The listing builds one solid part. Answer for the finished solid, in the listing's coordinates (mm). Face numbers are marked on the shaded views. Coordinates: 2 decimals unless noted, no trailing zeros. Order: outer loops, then holes, each group sorted by start corner. A loop starts at its lowest first (then second) coordinate and runs counter-clockwise, first axis right, second up. Notation, with made-up numbers: (-13, 78.5) - (42, 78.5) arc R17 cw to (42, 95.5) - close; hole circle Ø9 at (47, 11). An arc over 180 degrees is marked (long way). Use a Markdown table: item, result. Add a question column.
Item 1: The part is cut by section C-C, the plane y = 3.9. Give the vertices of the cut face in (x, z).
Item 2: The part is cut by section D-D, the plane x = -13.5. Give the vertices of the cut face in (y, z).
Item 3: Find the intervals of material crossed by line 1 along Y through (x, z) = (13, -1.75); line 2 along X through (y, z) = (4.85, 1); line 3 along Z through (x, y) = (1.5, 2.15), in increasing order.
Item 4: The mould has two halves that part along Z. Classify the marked faces 1, 2 and 3: released by +Z, released by -Z, zero draft, split by the parting line, or undercut.
Item 5: The part is cut by section A-A, the plane y = 1.5. State how many separate pieces and enclosed holes the cut face has, then the cut area to 3 significant figures.
Item 6: Flat-ended cylindrical pins translate along their axes: P1, Ø3, axis at x = -7.5, z = 0, coming from the -Y side; P2, Ø2.5, axis at x = 7.5, z = 0, coming from the +Y side; P3, Ø3, axis at y = 1.5, z = 2, coming from the +X side. Find the tip coordinate at first contact, or state that the pin passes through.
Item 7: The part is cut by section B-B, the plane x = 0. Give the vertices of the cut face in (y, z), then the cut area to 3 significant figures.
from build123d import *

# Parameters (mm, degrees)
BOSS_EXTRUDE1_DEPTH = 2
SKETCH2_R           = 4
SKETCH2_R_2         = 2.5
BOSS_EXTRUDE2_DEPTH = 3.5
SKETCH3_R           = 1.5
CUT_EXTRUDE1_DEPTH  = 5
SKETCH4_R           = 3
CUT_EXTRUDE2_DEPTH  = 1
SKETCH5_R           = 1
CUT_EXTRUDE3_DEPTH  = 5


with BuildPart() as part:
    # Sketch1 → Boss-Extrude1 (new body)
    with BuildSketch(Plane(origin=(0, 0, 0), x_dir=(1, 0, 0), z_dir=(0, 1, 0))):
        with BuildLine():
            Line((-16.5, 2.5), (-4.472135955, 4))
            ThreePointArc((-4.472135955, 4), (0, 6), (4.472135955, 4))
            Line((4.472135955, 4), (16.5, 2.5))
            ThreePointArc((16.5, 2.5), (19, 0), (16.5, -2.5))
            Line((16.5, -2.5), (4.472135955, -4))
            ThreePointArc((4.472135955, -4), (0, -6), (-4.472135955, -4))
            Line((-4.472135955, -4), (-16.5, -2.5))
            ThreePointArc((-16.5, -2.5), (-19, 0), (-16.5, 2.5))
        make_face()
    extrude(amount=BOSS_EXTRUDE1_DEPTH)

    # Sketch2 → Boss-Extrude2 (add)
    with BuildSketch(Plane(origin=(0, 2, 0), x_dir=(1, 0, 0), z_dir=(0, 1, 0))):
        with Locations(Location((0, 0, 0), (0, 0, 270))):
            Circle(SKETCH2_R)
        with Locations(Location((0, 0, 0), (0, 0, 270))):
            Circle(SKETCH2_R_2, mode=Mode.SUBTRACT)
    extrude(amount=BOSS_EXTRUDE2_DEPTH)

    # Sketch3 → Cut-Extrude1 (cut)
    with BuildSketch(Plane(origin=(0, 2, 0), x_dir=(1, 0, 0), z_dir=(0, 1, 0))):
        with Locations(Location((0, 0, 0), (0, 0, 270))):
            Circle(SKETCH3_R)
    extrude(amount=-CUT_EXTRUDE1_DEPTH, mode=Mode.SUBTRACT)

    # Sketch4 → Cut-Extrude2 (cut)
    with BuildSketch(Plane.XZ):
        with Locations(Location((0, 0, 0), (0, 0, 270))):
            Circle(SKETCH4_R)
    extrude(amount=-CUT_EXTRUDE2_DEPTH, mode=Mode.SUBTRACT)

    # Sketch5 → Cut-Extrude3 (cut)
    with BuildSketch(Plane.XZ):
        with Locations(Location((-16.5, 0, 0), (0, 0, 270))):
            Circle(SKETCH5_R)
        with Locations(Location((-10.5, 0, 0), (0, 0, 270))):
            Circle(SKETCH5_R)
        with Locations(Location((-7.5, 0, 0), (0, 0, 270))):
            Circle(SKETCH5_R)
        with Locations(Location((7.5, 0, 0), (0, 0, 270))):
            Circle(SKETCH5_R)
        with Locations(Location((10.5, 0, 0), (0, 0, 270))):
            Circle(SKETCH5_R)
        with Locations(Location((13.5, 0, 0), (0, 0, 270))):
            Circle(SKETCH5_R)
        with Locations(Location((16.5, 0, 0), (0, 0, 270))):
            Circle(SKETCH5_R)
        with Locations(Location((-13.5, 0, 0), (0, 0, 90))):
            Circle(SKETCH5_R)
    extrude(amount=-CUT_EXTRUDE3_DEPTH, mode=Mode.SUBTRACT)


solid = part.part
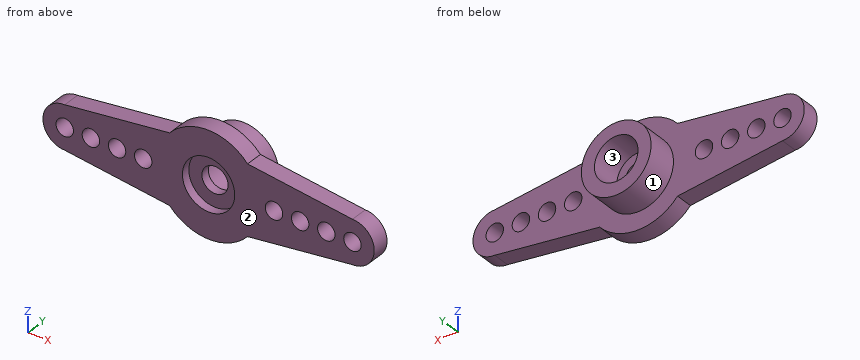
Solution:
| question | item | result |
|---|---|---|
| 1 | outline | circle Ø8 at (0, 0); hole circle Ø5 at (0, 0) |
| 2 | outline | (0, -2.87) - (2, -2.87) - (2, -1) - (0, -1) - close; (0, 1) - (2, 1) - (2, 2.87) - (0, 2.87) - close |
| 3 | line 1 | y = 0 to 2 |
| 3 | line 2 | x = -3.87 to -2.29, 2.29 to 3.87 |
| 3 | line 3 | z = -3.71 to -2, 2 to 3.71 |
| 4 | face 1 | split by the parting line |
| 4 | face 2 | zero draft |
| 4 | face 3 | undercut |
| 5 | separate pieces | 1 |
| 5 | enclosed holes | 9 |
| 5 | area | 240 mm2 |
| 6 | P1 | stops at y = 0 |
| 6 | P2 | stops at y = 2 |
| 6 | P3 | stops at x = 18.95 |
| 7 | outline | (0, -6) - (2, -6) - (2, -4) - (5.5, -4) - (5.5, -2.5) - (2, -2.5) - (2, -1.5) - (1, -1.5) - (1, -3) - (0, -3) - close; (0, 3) - (1, 3) - (1, 1.5) - (2, 1.5) - (2, 2.5) - (5.5, 2.5) - (5.5, 4) - (2, 4) - (2, 6) - (0, 6) - close |
| 7 | area | 25.5 mm2 |
